Could you check a few things on this model? Use its own coordinates, in mm. Face numbers are marked on the shaded views. A direction names the side the tool comes from. Give positions to 0.01 mm unless a question says otherwise; leave off trailing zeros. Loops run counter-clockwise (first coordinate to the right, second up) from the corner with the lowest first, then second, coordinate; pieces in that order, holes last.
1. Imagine slicing it at D-D (z = 8). List the corners of the cut face in (x, y) for me.
2. Imagine slicing it at C-C (y = 25.5). Count the separate pieces of the cut face and the enclosed holes in it, plus the area to 3 significant figures.
3. Thinking about a two-plate mould opening in Z: for the marked faces 1, 2 and 3, which applies, +Z half, -Z half, draft (parallel to the pull), parting line (faces both ways), or undercut?
4. For P1, Ø4.5, axis at x = -17.5, z = -57.8, coming from the -Y side; P2, Ø10, axis at y = 18, z = 25.5, coming from the -X side; P3, Ø1.5, axis at x = -11.5, y = 17.5, coming from the -Z side, each with a flat end and sliding along its axis, tell me the tip position at first contact or that it passes through.
5. Imagine slicing it at A-A (x = 0). List the corners of the cut face in (y, z) for me, plus the area to 3 significant figures.
6. I need wall thicknesses on line 1 along X through (y, z) = (19.5, -30.5); line 2 along X through (y, z) = (2, -52.5); line 3 along X through (y, z) = (12, 9). Which ranges of each line are inside material? Lowest first, please.
7. For the marked faces 4, 5, 6, 7 and 8, which set-ups out of +Z, -Z, +X, -X, +Y, -Y let a thin tool reach every point of the face, with its end or its side?
8. Imagine slicing it at B-B (z = -48). List the corners of the cut face in (x, y) for me, plus the area to 3 significant figures.
```python
from build123d import *

# Parameters (mm, degrees)
BOSS_EXTRUDE2_DEPTH = 27
BOSS_EXTRUDE3_DEPTH = 5
SKETCH6_R           = 3.75
BOSS_EXTRUDE8_DEPTH = 4
SKETCH3_R           = 1.5
CUT_EXTRUDE2_DEPTH  = 33
SKETCH7_R           = 3.75
BOSS_EXTRUDE9_DEPTH = 8
SKETCH8_R           = 3.75
CUT_EXTRUDE4_DEPTH  = 24
SKETCH9_R           = 1.375
CUT_EXTRUDE5_DEPTH  = 33
CUT_EXTRUDE6_DEPTH  = 2
SKETCH13_R          = 8
CUT_EXTRUDE8_DEPTH  = 122.75
CUT_EXTRUDE9_REACH  = 131.287
SKETCH14_R          = 8
CUT_EXTRUDE11_REACH = 105.053
SKETCH16_R          = 8
CUT_EXTRUDE12_REACH = 131.287
SKETCH17_R          = 8
CUT_EXTRUDE13_REACH = 121.393
SKETCH19_R          = 8
CUT_EXTRUDE14_REACH = 121.393
SKETCH20_R          = 8
SKETCH21_R          = 8
SKETCH21_W          = 16
SKETCH21_H          = 13
CUT_EXTRUDE15_DEPTH = 3
SKETCH22_W          = 16
SKETCH22_H          = 13
CUT_EXTRUDE16_DEPTH = 9.75


with BuildPart() as part:
    # Sketch1 → Boss-Extrude2 (new body)
    with BuildSketch(Plane(origin=(0, 0, 0), x_dir=(1, 0, 0), z_dir=(0, 1, 0))):
        Polygon((-43.178681761, 29.873916914), (-17.5, 45.604089113), (-17.5, 57.803420417), (17.5, 57.803420417), (17.5, 45.604089113), (43.178681761, 29.873916914), (59, 2.406681305), (59, -41.5), (-59, -41.5), (-59, 2.406681305), align=None)
        Polygon((39.481402229, 26.275231503), (12.5, 42.803420417), (12.5, 52.803420417), (-12.5, 52.803420417), (-12.5, 42.803420417), (-39.481402229, 26.275231503), (-54, 1.069636136), (-54, -36.5), (54, -36.5), (54, 1.069636136), align=None, mode=Mode.SUBTRACT)
    extrude(amount=BOSS_EXTRUDE2_DEPTH)

    # Sketch2 → Boss-Extrude3 (add)
    with BuildSketch(Plane.XZ):
        Polygon((17.5, -57.803420417), (-17.5, -57.803420417), (-17.5, -45.604089113), (-43.178681761, -29.873916914), (-59, -2.406681305), (-59, 41.5), (59, 41.5), (59, -2.406681305), (43.178681761, -29.873916914), (17.5, -45.604089113), align=None)
    extrude(amount=BOSS_EXTRUDE3_DEPTH)

    # Sketch6 → Boss-Extrude8 (add)
    with BuildSketch(Plane(origin=(0, 0, 0), x_dir=(1, 0, 0), z_dir=(0, 1, 0))):
        with Locations((-19.63, 13.76)):
            Circle(SKETCH6_R)
        with Locations((-36.69, -20.73)):
            Circle(SKETCH6_R)
        with Locations((23.64, 0.27)):
            Circle(SKETCH6_R)
        with Locations((45.36, -27.86)):
            Circle(SKETCH6_R)
    extrude(amount=BOSS_EXTRUDE8_DEPTH)

    # Sketch3 → Cut-Extrude2 (cut, through all)
    with BuildSketch(Plane(origin=(0, -5, 0), x_dir=(-1, 0, 0), z_dir=(0, -1, 0))):
        with Locations((-45.36, -27.86)):
            Circle(SKETCH3_R)
        with Locations((-23.64, 0.27)):
            Circle(SKETCH3_R)
        with Locations((19.63, 13.76)):
            Circle(SKETCH3_R)
        with Locations((36.69, -20.73)):
            Circle(SKETCH3_R)
    extrude(amount=-CUT_EXTRUDE2_DEPTH, mode=Mode.SUBTRACT)

    # Sketch7 → Boss-Extrude9 (add)
    with BuildSketch(Plane(origin=(0, 27, 0), x_dir=(1, 0, 0), z_dir=(0, 1, 0))):
        with Locations((-59, -41.5)):
            Circle(SKETCH7_R)
        with Locations((-59, 2.406681305)):
            Circle(SKETCH7_R)
        with Locations((-43.178681761, 29.873916914)):
            Circle(SKETCH7_R)
        with Locations((-17.5, 57.803420417)):
            Circle(SKETCH7_R)
        with Locations((17.5, 57.803420417)):
            Circle(SKETCH7_R)
        with Locations((43.178681761, 29.873916914)):
            Circle(SKETCH7_R)
        with Locations((59, 2.406681305)):
            Circle(SKETCH7_R)
        with Locations((59, -41.5)):
            Circle(SKETCH7_R)
    extrude(amount=-BOSS_EXTRUDE9_DEPTH)

    # Sketch8 → Cut-Extrude4 (cut)
    with BuildSketch(Plane.XZ.offset(5)):
        with Locations((59, 41.5)):
            Circle(SKETCH8_R)
        with Locations((59, -2.406681305)):
            Circle(SKETCH8_R)
        with Locations((43.178681761, -29.873916914)):
            Circle(SKETCH8_R)
        with Locations((17.5, -57.803420417)):
            Circle(SKETCH8_R)
        with Locations((-17.5, -57.803420417)):
            Circle(SKETCH8_R)
        with Locations((-43.178681761, -29.873916914)):
            Circle(SKETCH8_R)
        with Locations((-59, -2.406681305)):
            Circle(SKETCH8_R)
        with Locations((-59, 41.5)):
            Circle(SKETCH8_R)
    extrude(amount=-CUT_EXTRUDE4_DEPTH, mode=Mode.SUBTRACT)

    # Sketch9 → Cut-Extrude5 (cut, through all)
    with BuildSketch(Plane(origin=(0, 27, 0), x_dir=(1, 0, 0), z_dir=(0, 1, 0))):
        with Locations((-59, -41.5)):
            Circle(SKETCH9_R)
        with Locations((-59, 2.406681305)):
            Circle(SKETCH9_R)
        with Locations((-17.5, 57.803420417)):
            Circle(SKETCH9_R)
        with Locations((43.178681761, 29.873916914)):
            Circle(SKETCH9_R)
        with Locations((17.5, 57.803420417)):
            Circle(SKETCH9_R)
        with Locations((-43.178681761, 29.873916914)):
            Circle(SKETCH9_R)
        with Locations((59, 2.406681305)):
            Circle(SKETCH9_R)
        with Locations((59, -41.5)):
            Circle(SKETCH9_R)
    extrude(amount=-CUT_EXTRUDE5_DEPTH, mode=Mode.SUBTRACT)

    # Sketch11 → Cut-Extrude6 (cut)
    with BuildSketch(Plane(origin=(0, 0, 0), x_dir=(1, 0, 0), z_dir=(0, 1, 0))):
        Polygon((27.5, -36.5), (27.5, -6.5), (12.5, -6.5), (12.5, 38.5), (-12.5, 38.5), (-12.5, -6.5), (-27.5, -6.5), (-27.5, -36.5), align=None)
    extrude(amount=-CUT_EXTRUDE6_DEPTH, mode=Mode.SUBTRACT)

    # Sketch13 → Cut-Extrude8 (cut, through all)
    with BuildSketch(Plane.ZY.offset(59)):
        with Locations((13.343318695, 27)):
            Circle(SKETCH13_R)
    extrude(amount=-CUT_EXTRUDE8_DEPTH, mode=Mode.SUBTRACT)

    # Sketch14 → Cut-Extrude9 (cut, up to next)
    with BuildSketch(Plane(origin=(-45.342387005, 0, -26.117529435), x_dir=(-0.499126718, 0, 0.866529006), z_dir=(-0.866529006, 0, -0.499126718)), mode=Mode.PRIVATE) as cut_extrude9_sk1:
        with Locations((11.514017709, 27)):
            Circle(SKETCH14_R)
    cut_extrude9_tool1 = extrude(cut_extrude9_sk1.sketch, amount=-CUT_EXTRUDE9_REACH, mode=Mode.PRIVATE) & part.part
    add(cut_extrude9_tool1.solids().sort_by_distance((-51.089341, 27, -16.140299))[0], mode=Mode.SUBTRACT)

    # Sketch16 → Cut-Extrude11 (cut, up to next)
    with BuildSketch(Plane(origin=(0, 0, -57.803420417), x_dir=(-1, 0, 0), z_dir=(0, 0, -1)), mode=Mode.PRIVATE) as cut_extrude11_sk1:
        with Locations((0, 27)):
            Circle(SKETCH16_R)
    cut_extrude11_tool1 = extrude(cut_extrude11_sk1.sketch, amount=-CUT_EXTRUDE11_REACH, mode=Mode.PRIVATE) & part.part
    add(cut_extrude11_tool1.solids().sort_by_distance((0, 27, -57.80342))[0], mode=Mode.SUBTRACT)

    # Sketch17 → Cut-Extrude12 (cut, up to next)
    with BuildSketch(Plane(origin=(45.342387005, 0, -26.117529435), x_dir=(-0.499126718, 0, -0.866529006), z_dir=(0.866529006, 0, -0.499126718)), mode=Mode.PRIVATE) as cut_extrude12_sk1:
        with Locations((-11.514017709, 27)):
            Circle(SKETCH17_R)
    cut_extrude12_tool1 = extrude(cut_extrude12_sk1.sketch, amount=-CUT_EXTRUDE12_REACH, mode=Mode.PRIVATE) & part.part
    add(cut_extrude12_tool1.solids().sort_by_distance((51.089341, 27, -16.140299))[0], mode=Mode.SUBTRACT)

    # Sketch19 → Cut-Extrude13 (cut, up to next)
    with BuildSketch(Plane(origin=(-25.088449392, 0, -40.955578852), x_dir=(-0.852725133, 0, 0.522359882), z_dir=(-0.522359882, 0, -0.852725133)), mode=Mode.PRIVATE) as cut_extrude13_sk1:
        with Locations((4.464611438, 27)):
            Circle(SKETCH19_R)
    cut_extrude13_tool1 = extrude(cut_extrude13_sk1.sketch, amount=-CUT_EXTRUDE13_REACH, mode=Mode.PRIVATE) & part.part
    add(cut_extrude13_tool1.solids().sort_by_distance((-28.895536, 27, -38.623445))[0], mode=Mode.SUBTRACT)

    # Sketch20 → Cut-Extrude14 (cut, up to next)
    with BuildSketch(Plane(origin=(25.088449392, 0, -40.955578852), x_dir=(-0.852725133, 0, -0.522359882), z_dir=(0.522359882, 0, -0.852725133)), mode=Mode.PRIVATE) as cut_extrude14_sk1:
        with Locations((-4.464611438, 27)):
            Circle(SKETCH20_R)
    cut_extrude14_tool1 = extrude(cut_extrude14_sk1.sketch, amount=-CUT_EXTRUDE14_REACH, mode=Mode.PRIVATE) & part.part
    add(cut_extrude14_tool1.solids().sort_by_distance((28.895536, 27, -38.623445))[0], mode=Mode.SUBTRACT)

    # Sketch21 → Cut-Extrude15 (cut)
    with BuildSketch(Plane(origin=(0, 0, 36.5), x_dir=(-1, 0, 0), z_dir=(0, 0, -1))):
        with Locations((38, 27)):
            Circle(SKETCH21_R)
        with Locations((-24, 12.5)):
            Rectangle(SKETCH21_W, SKETCH21_H)
    extrude(amount=-CUT_EXTRUDE15_DEPTH, mode=Mode.SUBTRACT)

    # Sketch22 → Cut-Extrude16 (cut, through all)
    with BuildSketch(Plane(origin=(0, 0, 36.5), x_dir=(-1, 0, 0), z_dir=(0, 0, -1))):
        with Locations((16, 12.5)):
            Rectangle(SKETCH22_W, SKETCH22_H)
    extrude(amount=-CUT_EXTRUDE16_DEPTH, mode=Mode.SUBTRACT)


solid = part.part
```
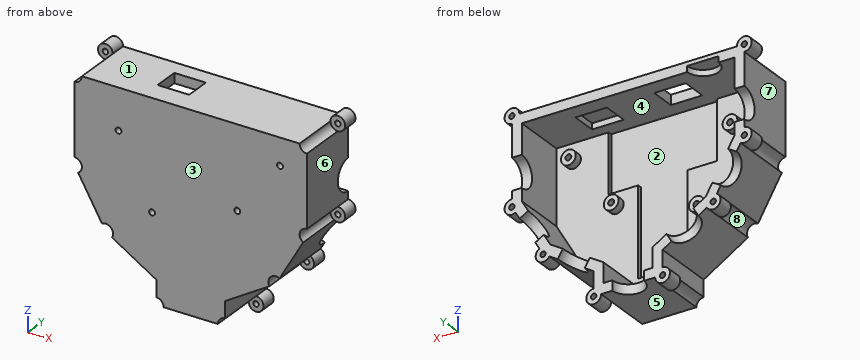
Derived:
1. outline: (-59, -5) - (59, -5) - (59, 21.05) - (54, 21.05) - (54, 0) - (27.5, 0) - (27.5, -2) - (-27.5, -2) - (-27.5, 0) - (-54, 0) - (-54, 21.05) - (-59, 21.05) - close
2. separate pieces: 7
2. enclosed holes: 8
2. area: 1,440 mm2
3. face 1: +Z half
3. face 2: undercut
3. face 3: draft
4. P1: stops at y = 19
4. P2: stops at x = -59
4. P3: stops at z = -57.8
5. outline: (-5, -57.8) - (19, -57.8) - (19, -52.8) - (0, -52.8) - (0, -38.5) - (-2, -38.5) - (-2, 36.5) - (27, 36.5) - (27, 41.5) - (-5, 41.5) - close
5. area: 577 mm2
6. line 1: x = -46.88 to -44.4, -41.95 to -32.58, 32.58 to 41.95, 44.4 to 46.88
6. line 2: x = -17.5 to -12.5, 12.5 to 17.5
6. line 3: x = -59 to -54, 54 to 59
7. face 4: +Y
7. face 5: -Z, +Y, -Y
7. face 6: +X, +Y, -Y
7. face 7: -X, +Y, -Y
7. face 8: -Y
8. outline: (-17.5, -5) - (17.5, -5) - (17.5, 27) - (12.5, 27) - (12.5, 0) - (-12.5, 0) - (-12.5, 27) - (-17.5, 27) - close
8. area: 445 mm2
